from build123d import *

# Parameters (mm, degrees)
F1_DEPTH = 2
F2_R     = 2
F3_DEPTH = 2
F2_R_2   = 3
F4_DEPTH = 1
F5_SIZE  = 1


with BuildPart() as f1:
    # F0 (on Top) → F1 (new body)
    with BuildSketch(Plane.XY):
        with BuildLine():
            ThreePointArc((32.5, 27.5), (31.035534, 31.035534), (27.5, 32.5))
            Line((27.5, 32.5), (-27.5, 32.5))
            ThreePointArc((-27.5, 32.5), (-31.035534, 31.035534), (-32.5, 27.5))
            Line((-32.5, 27.5), (-32.5, -27.5))
            ThreePointArc((-32.5, -27.5), (-31.035534, -31.035534), (-27.5, -32.5))
            Line((-27.5, -32.5), (27.5, -32.5))
            ThreePointArc((27.5, -32.5), (31.035534, -31.035534), (32.5, -27.5))
            Line((32.5, -27.5), (32.5, 27.5))
        make_face()
    extrude(amount=F1_DEPTH)

    # F2 (on face) → F3 (cut, through all)
    with BuildSketch(Plane.XY.offset(2)):
        with Locations((-27.5, 27.5)):
            Circle(F2_R)
        with Locations((27.5, 27.5)):
            Circle(F2_R)
        with Locations((27.5, -27.5)):
            Circle(F2_R)
        with Locations((-27.5, -27.5)):
            Circle(F2_R)
    extrude(amount=-F3_DEPTH, mode=Mode.SUBTRACT)

    # F2 (on face) → F4 (cut)
    with BuildSketch(Plane.XY.offset(2)):
        with Locations((-27.5, 27.5)):
            Circle(F2_R_2)
        with Locations((-27.5, 27.5)):
            Circle(F2_R, mode=Mode.SUBTRACT)
        with Locations((27.5, 27.5)):
            Circle(F2_R_2)
        with Locations((27.5, 27.5)):
            Circle(F2_R, mode=Mode.SUBTRACT)
        with Locations((-27.5, -27.5)):
            Circle(F2_R_2)
        with Locations((-27.5, -27.5)):
            Circle(F2_R, mode=Mode.SUBTRACT)
        with Locations((27.5, -27.5)):
            Circle(F2_R_2)
        with Locations((27.5, -27.5)):
            Circle(F2_R, mode=Mode.SUBTRACT)
    extrude(amount=-F4_DEPTH, mode=Mode.SUBTRACT)

    # F5
    f5_edges = [f1.edges().sort_by_distance(p)[0] for p in [
        (-32.5, 0, 2),
        (-31.035534, 31.035534, 2),
        (0, 32.5, 2),
        (31.035534, 31.035534, 2),
        (32.5, 0, 2),
        (31.035534, -31.035534, 2),
        (0, -32.5, 2),
        (-31.035534, -31.035534, 2),
    ]]
    chamfer(f5_edges, length=F5_SIZE)


solid = f1.part
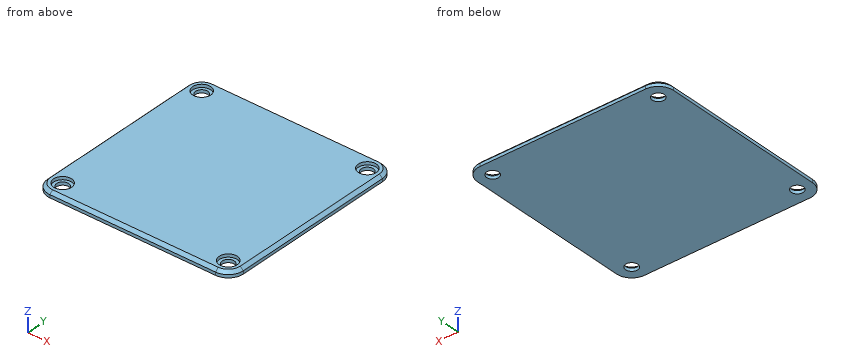
Design review of the part built by this model. Coordinates are the model's own, in mm. Round coordinates to 2 decimals unless told otherwise and drop trailing zeros. Write each loop counter-clockwise with the first axis right and the second up, starting at its lowest first coordinate (ties: lowest second). Pieces come first, ordered by that corner, then holes. Notation, with made-up numbers: M 5.5,73.25 L 24.5,73.25 A28 ccw 24.5,112.25 Z; hole C 83.5,-34 d10. An arc over 180 degrees is marked long. One line per item, written item: value. Start each with the question number.
1. Take a section at A-A on z = 0.45. State the section outline as (x, y) points.
2. To check wall thickness, follow probe 1 along Y at (x, z) = (-27.5, 0.4); probe 2 along Y at (x, z) = (26, 0.8); probe 3 along X at (y, z) = (29, 0.8). State the ranges of each line that lie inside material, in increasing order. Write a range as from..to.
3. Clearance check with a flat-ended pin moving along its axis: P1, Ø3, axis at x = 28, y = 28.5, coming from the +Z side. State where the tip first meets the part, or that it passes through.
Computed:
1. outline: M -32.5,-27.5 A5 ccw -27.5,-32.5 L 27.5,-32.5 A5 ccw 32.5,-27.5 L 32.5,27.5 A5 ccw 27.5,32.5 L -27.5,32.5 A5 ccw -32.5,27.5 Z; hole C -27.5,-27.5 d4; hole C -27.5,27.5 d4; hole C 27.5,-27.5 d4; hole C 27.5,27.5 d4
2. probe 1: y = -32.5..-29.5, -25.5..25.5, 29.5..32.5
2. probe 2: y = -32.5..-28.82, -26.18..26.18, 28.82..32.5
2. probe 3: x = -32.27..-28.82, -26.18..26.18, 28.82..32.27
3. P1: stops at z = 1
